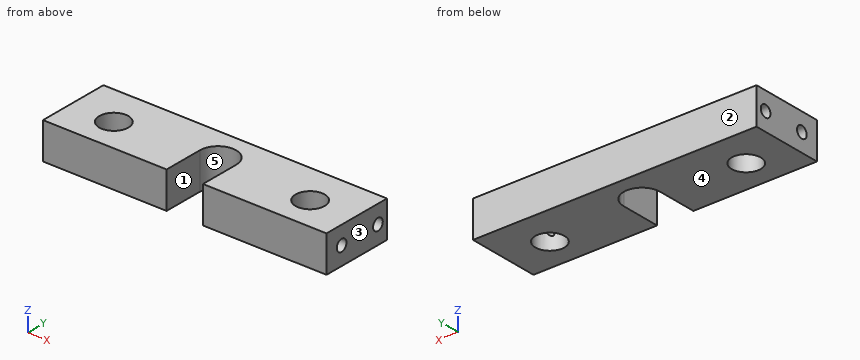
from build123d import *

# Parameters (mm, degrees)
SKETCH1_W                       = 5
SKETCH1_H                       = 10
BOSS_EXTRUDE1_DEPTH             = 39
TAP_DRILL_FOR_M2X0_4_TAP1_D     = 1.6
TAP_DRILL_FOR_M2X0_4_TAP1_DEPTH = 5
TAP_DRILL_FOR_M2X0_4_TAP1_TIP   = 0.480688495
TAP_DRILL_FOR_M2X0_4_TAP2_D     = 1.6
TAP_DRILL_FOR_M2X0_4_TAP2_DEPTH = 5
TAP_DRILL_FOR_M2X0_4_TAP2_TIP   = 0.480688495
CUT_EXTRUDE1_REACH              = 7
SKETCH8_R                       = 2


with BuildPart() as part:
    # Sketch1 → Boss-Extrude1 (new body)
    with BuildSketch(Plane(origin=(0, 0, 0), x_dir=(0, 0, -1), z_dir=(1, 0, 0))):
        with Locations((0, 5)):
            Rectangle(SKETCH1_W, SKETCH1_H)
    extrude(amount=BOSS_EXTRUDE1_DEPTH)

    # Tap Drill for M2x0.4 Tap1
    with Locations(Plane(origin=(39, 0, 0), x_dir=(0, 0, -1), z_dir=(1, 0, 0))):
        with Locations((0, 8.5), (0, 2.5)):
            Hole(TAP_DRILL_FOR_M2X0_4_TAP1_D / 2, depth=TAP_DRILL_FOR_M2X0_4_TAP1_DEPTH)
            with Locations((0, 0, -(TAP_DRILL_FOR_M2X0_4_TAP1_DEPTH + TAP_DRILL_FOR_M2X0_4_TAP1_TIP / 2))):  # 118° drill point
                Cone(0, TAP_DRILL_FOR_M2X0_4_TAP1_D / 2, TAP_DRILL_FOR_M2X0_4_TAP1_TIP, mode=Mode.SUBTRACT)

    # Tap Drill for M2x0.4 Tap2
    with Locations(Plane.ZY):
        with Locations((0, 8.5), (0, 2.5)):
            Hole(TAP_DRILL_FOR_M2X0_4_TAP2_D / 2, depth=TAP_DRILL_FOR_M2X0_4_TAP2_DEPTH)
            with Locations((0, 0, -(TAP_DRILL_FOR_M2X0_4_TAP2_DEPTH + TAP_DRILL_FOR_M2X0_4_TAP2_TIP / 2))):  # 118° drill point
                Cone(0, TAP_DRILL_FOR_M2X0_4_TAP2_D / 2, TAP_DRILL_FOR_M2X0_4_TAP2_TIP, mode=Mode.SUBTRACT)

    # Sketch8 → Cut-Extrude1 (cut, up to next)
    with BuildSketch(Plane.XY.offset(2.5), mode=Mode.PRIVATE) as cut_extrude1_sk1:
        with Locations((6, 4.5)):
            Circle(SKETCH8_R)
    cut_extrude1_tool1 = extrude(cut_extrude1_sk1.sketch, amount=-CUT_EXTRUDE1_REACH, mode=Mode.PRIVATE) & part.part
    add(cut_extrude1_tool1.solids().sort_by_distance((6, 4.5, 2.5))[0], mode=Mode.SUBTRACT)
    # Sketch8 → Cut-Extrude1 (cut, up to next)
    with BuildSketch(Plane.XY.offset(2.5), mode=Mode.PRIVATE) as cut_extrude1_sk2:
        with Locations((33, 4.5)):
            Circle(SKETCH8_R)
    cut_extrude1_tool2 = extrude(cut_extrude1_sk2.sketch, amount=-CUT_EXTRUDE1_REACH, mode=Mode.PRIVATE) & part.part
    add(cut_extrude1_tool2.solids().sort_by_distance((33, 4.5, 2.5))[0], mode=Mode.SUBTRACT)
    # Sketch8 → Cut-Extrude1 (cut, up to next)
    with BuildSketch(Plane.XY.offset(2.5), mode=Mode.PRIVATE) as cut_extrude1_sk3:
        with BuildLine():
            Line((17, 0), (17, 5.5))
            ThreePointArc((17, 5.5), (19.5, 8), (22, 5.5))
            Line((22, 5.5), (22, 0))
            Line((22, 0), (17, 0))
        make_face()
    cut_extrude1_tool3 = extrude(cut_extrude1_sk3.sketch, amount=-CUT_EXTRUDE1_REACH, mode=Mode.PRIVATE) & part.part
    add(cut_extrude1_tool3.solids().sort_by_distance((19.5, 3.752606, 2.5))[0], mode=Mode.SUBTRACT)


solid = part.part
Geometry: final body of the model. Coordinates: model frame, mm. Face numbers are marked on the shaded views. A direction names the side the tool comes from. Give positions to 0.01 mm unless a question says otherwise; leave off trailing zeros. Write each loop counter-clockwise with the first axis right and the second up, starting at its lowest first coordinate (ties: lowest second). Pieces come first, ordered by that corner, then holes. Notation, with made-up numbers: M -14,49.25 L 10,49.25 A21 ccw 10,56.25 Z; hole C 47,-18 d5. An arc over 180 degrees is marked long. Answer in a Markdown table with one row per item. Add a question column.
(1) Section C-C on x = 32.5. Return loops of the section in (y, z).
(2) Section B-B on z = 1.15. Return loops of the section in (x, y), and give its area (3 significant figures).
(3) Reachability of the marked faces 1 and 2 from +Z, -Z, +X, -X, +Y, -Y: full face, straight path, thin tool, end or side. Return the list, or none.
(4) First-contact query: pin 1 (1.4 mm diameter, centred on y = 8.5, z = 0, fed in from +X); pin 2 (1.5 mm diameter, centred on y = 8.5, z = 0, fed in from -X). Flat tips, straight axial feed; report the tip coordinate or a pass-through.
(5) Mould query, pull axis X, two halves, no side actions, for the marked faces 3, 4 and 5. Classes: +X half, -X half, draft (parallel to the pull), parting line (faces both ways), or undercut.
(6) Section D-D on x = 7. Return loops of the section in (y, z), and give its area (3 significant figures).
(7) Ray query, line 1 (Y direction, x = 35.1, z = 0); line 2 (Z direction, x = 3.2, y = 8.5); line 3 (X direction, y = 5, z = -0.1). Return the intervals inside material, ascending.
(8) Section A-A on y = 4.5. Return loops of the section in (x, z).
Result set:
| question | item | result |
|---|---|---|
| 1 | outline | M 0,-2.5 L 2.56,-2.5 L 2.56,2.5 L 0,2.5 Z; M 6.44,-2.5 L 10,-2.5 L 10,2.5 L 6.44,2.5 Z |
| 2 | outline | M 0,0 L 17,0 L 17,5.5 A2.5 cw 22,5.5 L 22,0 L 39,0 L 39,10 L 0,10 Z; hole C 6,4.5 d4; hole C 33,4.5 d4 |
| 2 | area | 328 mm^2 |
| 3 | face 1 | +Z, -Z, -Y |
| 3 | face 2 | +Z, -Z, +X, -X, +Y |
| 4 | pin 1 | stops at x = 33.94 |
| 4 | pin 2 | stops at x = 5.03 |
| 5 | face 3 | +X half |
| 5 | face 4 | draft |
| 5 | face 5 | undercut |
| 6 | outline | M 0,-2.5 L 2.77,-2.5 L 2.77,2.5 L 0,2.5 Z; M 6.23,-2.5 L 10,-2.5 L 10,2.5 L 6.23,2.5 Z |
| 6 | area | 32.7 mm^2 |
| 7 | line 1 | y = 0 to 1.7, 3.3 to 7.7, 9.3 to 10 |
| 7 | line 2 | z = -2.5 to -0.8, 0.8 to 2.5 |
| 7 | line 3 | x = 0 to 4.06, 7.94 to 17, 22 to 31.06, 34.94 to 39 |
| 8 | outline | M 0,-2.5 L 4,-2.5 L 4,2.5 L 0,2.5 Z; M 8,-2.5 L 17,-2.5 L 17,2.5 L 8,2.5 Z; M 22,-2.5 L 31,-2.5 L 31,2.5 L 22,2.5 Z; M 35,-2.5 L 39,-2.5 L 39,2.5 L 35,2.5 Z |
